from build123d import *
from build123d.topology import SkipClean

# Parameters (mm, degrees)
SKETCH_1_R      = 2.85
SKETCH_1_R_2    = 1.25
EXTRUDE_1_DEPTH = 0.9
EXTRUDE_2_DEPTH = 0.5


with BuildPart() as part:
    # ｽｹｯﾁ1 → ﾎﾞｽ - 押し出し1 (new body)
    with BuildSketch(Plane.XY):
        Circle(SKETCH_1_R)
        Circle(SKETCH_1_R_2, mode=Mode.SUBTRACT)
    extrude_1 = extrude(amount=EXTRUDE_1_DEPTH)

    # ｽｹｯﾁ2 → ﾎﾞｽ - 押し出し2 (add)
    with SkipClean():  # the faces are left unmerged after this step: merging them gives an invalid solid
        with BuildSketch(Plane.XY.offset(0.9)):
            with BuildLine():
                Line((-1, 2.668801229), (-1, 1.789553017))
                ThreePointArc((-1, 1.789553017), (-2.05, 0), (-1, -1.789553017))
                Line((-1, -1.789553017), (-1, -2.668801229))
                ThreePointArc((-1, -2.668801229), (-2.85, 0), (-1, 2.668801229))
            make_face()
            with BuildLine():
                Line((1, 2.668801229), (1, 1.789553017))
                ThreePointArc((1, 1.789553017), (2.05, 0), (1, -1.789553017))
                Line((1, -1.789553017), (1, -2.668801229))
                ThreePointArc((1, -2.668801229), (2.85, 0), (1, 2.668801229))
            make_face()
        extrude_2 = extrude(amount=EXTRUDE_2_DEPTH)

    # ﾐﾗｰ1: ﾎﾞｽ - 押し出し1, ﾎﾞｽ - 押し出し2 across plane
    with SkipClean():  # the faces are left unmerged after this step: merging them gives an invalid solid
        add(extrude_1.mirror(Plane.XY))
        add(extrude_2.mirror(Plane.XY))


solid = part.part
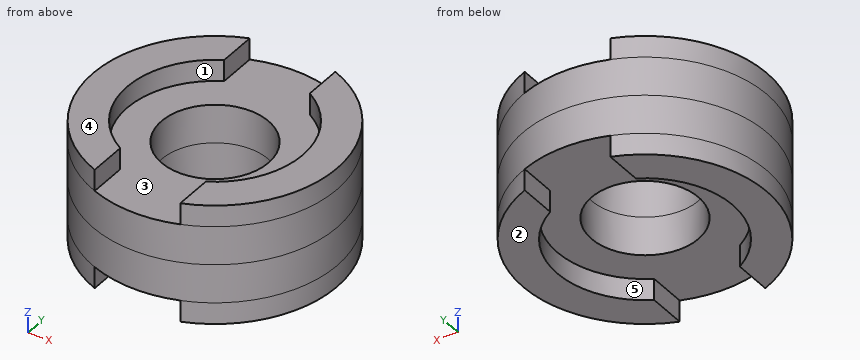
Verification items for the finished model (mm, model axes). Face numbers are marked on the shaded views. A direction names the side the tool comes from. Coordinates: 2 decimals unless noted, no trailing zeros. Order: outer loops, then holes, each group sorted by start corner. A loop starts at its lowest first (then second) coordinate and runs counter-clockwise, first axis right, second up.
1. Release check for a two-part mould opening along X. For the marked faces 1 and 2 record: +X half, -X half, draft (parallel to the pull), parting line (faces both ways), or undercut.
Results found:
face 1: undercut
face 2: draft
2. Scan lines: line 1 (Y direction, x = 0, z = 0.4); line 2 (X direction, y = 1, z = 1.25); line 3 (Z direction, x = 0.9, y = -2.15). Record each from-to range of solid material in increasing order.
Results found:
line 1: y = -2.85 to -1.25, 1.25 to 2.85
line 2: x = -2.67 to -1.79, 1.79 to 2.67
line 3: z = -0.9 to 0.9
3. Go/stop test with flat-tipped pins: pin 1 Ø3 at (x, y) = (0, 0) entering from +Z; pin 2 Ø0.5 at (y, z) = (2, -1) entering from -X; pin 3 Ø2 at (x, y) = (0, 0) entering from +Z; pin 4 Ø0.5 at (y, z) = (-2, -1) entering from +X. Record where each tip stops, or that it passes through.
Results found:
pin 1: stops at z = 0.9
pin 2: stops at x = -2.25
pin 3: passes through
pin 4: stops at x = 2.25
4. Sectioned sample at A-A, the plane z = 1.2. Record the cut outline in (x, y), and give its area (3 significant figures).
Results found:
outline: (-1, -2.67) - (-1, -1.79) arc R2.05 cw to (-1, 1.79) - (-1, 2.67) arc R2.85 ccw to start; (1, -2.67) arc R2.85 ccw to (1, 2.67) - (1, 1.79) arc R2.05 cw to (1, -1.79) - close
area: 9.02 mm2
5. Sectioned sample at C-C, the plane x = 0. Record the cut outline in (y, z), and give its area (3 significant figures).
Results found:
outline: (-2.85, -0.9) - (-1.25, -0.9) - (-1.25, 0.9) - (-2.85, 0.9) - close; (1.25, -0.9) - (2.85, -0.9) - (2.85, 0.9) - (1.25, 0.9) - close
area: 5.76 mm2
6. Sectioned sample at B-B, the plane y = 0. Record the cut outline in (x, z), and give its area (3 significant figures).
Results found:
outline: (-2.85, -1.4) - (-2.05, -1.4) - (-2.05, -0.9) - (-1.25, -0.9) - (-1.25, 0.9) - (-2.05, 0.9) - (-2.05, 1.4) - (-2.85, 1.4) - close; (1.25, -0.9) - (2.05, -0.9) - (2.05, -1.4) - (2.85, -1.4) - (2.85, 1.4) - (2.05, 1.4) - (2.05, 0.9) - (1.25, 0.9) - close
area: 7.36 mm2
7. Sectioned sample at D-D, the plane y = 1. Record the cut outline in (x, z).
Results found:
outline: (-2.67, -1.4) - (-1.79, -1.4) - (-1.79, -0.9) - (-0.75, -0.9) - (-0.75, 0.9) - (-1.79, 0.9) - (-1.79, 1.4) - (-2.67, 1.4) - close; (0.75, -0.9) - (1.79, -0.9) - (1.79, -1.4) - (2.67, -1.4) - (2.67, 1.4) - (1.79, 1.4) - (1.79, 0.9) - (0.75, 0.9) - close
8. Set-up check for the marked faces 3, 4 and 5: record each of +Z, -Z, +X, -X, +Y, -Y from which the full face is reachable in a straight line by a thin tool's end or side.
Results found:
face 3: +Z
face 4: +Z, +X, -X, +Y, -Y
face 5: -Z
